Read the model definition and answer for the solid it produces. Units are mm, in the model's axes. Face numbers are marked on the shaded views. A direction names the side the tool comes from. Coordinates: 2 decimals unless noted, no trailing zeros. Order: outer loops, then holes, each group sorted by start corner. A loop starts at its lowest first (then second) coordinate and runs counter-clockwise, first axis right, second up. Notation, with made-up numbers: (74.5, 31.5) -> (97.5, 31.5) arc R34 cw to (97.5, 69.5) -> close; hole circle Ø4 at (6.25, -23). An arc over 180 degrees is marked (long way). Answer in a Markdown table with one row per item.
from build123d import *

# Parameters (mm, degrees)
F0_W     = 425.45
F0_H     = 283.972
F1_DEPTH = 101.6
F3_DEPTH = 41.275
F2_W     = 12.7
F2_H     = 69.85
F4_DEPTH = 44.45
F6_DEPTH = 12.7


with BuildPart() as f1:
    # F0 (on Top) → F1 (new body)
    with BuildSketch(Plane.XY):
        Rectangle(F0_W, F0_H)
    extrude(amount=F1_DEPTH)

    # F2 (on face) → F3 (cut)
    with BuildSketch(Plane.XY.offset(101.6)):
        with BuildLine():
            Line((104.775, 57.15), (104.775, 44.45))
            Line((104.775, 44.45), (-104.775, 44.45))
            Line((-104.775, 44.45), (-104.775, 57.15))
            Line((-104.775, 57.15), (-119.0752, 57.15))
            Line((-119.0752, 57.15), (-119.0752, 88.9))
            Line((-119.0752, 88.9), (-111.125, 88.9))
            Line((-111.125, 88.9), (-111.125, 95.25))
            Line((-111.125, 95.25), (-136.525, 95.25))
            Line((-136.525, 95.25), (-136.525, 88.9))
            Line((-136.525, 88.9), (-128.5748, 88.9))
            Line((-128.5748, 88.9), (-128.5748, 57.15))
            Line((-128.5748, 57.15), (-142.875, 57.15))
            Line((-142.875, 57.15), (-142.875, 34.925))
            Line((-142.875, 34.925), (-98.425, 34.925))
            Line((-98.425, 34.925), (-98.425, -58.3184))
            Line((-98.425, -58.3184), (-34.925, -58.3184))
            Line((-34.925, -58.3184), (0.6356468836, -93.881381557))
            Line((0.6356468836, -93.881381557), (23.5001294705, -71.0184))
            Line((23.5001294705, -71.0184), (40.6451294705, -71.0184))
            Line((40.6451294705, -71.0184), (40.6451294705, -83.7184))
            add(Edge.make_bspline(
                [(98.425, -95.25), (85.7012200048, -95.9646103609), (83.2737472807, -107.5863293593), (52.6561842817, -111.0807364969), (41.7633484197, -97.2699226213), (41.6022054851, -92.9006263614), (40.6451294705, -83.7184)],
                knots=[0, 0, 0, 0, 0.2714742221, 0.5613518333, 0.7763996456, 1, 1, 1, 1], degree=3))
            Line((98.425, -95.25), (98.425, 34.925))
            Line((98.425, 34.925), (142.875, 34.925))
            Line((142.875, 34.925), (142.875, 57.15))
            Line((142.875, 57.15), (128.5748, 57.15))
            Line((128.5748, 57.15), (128.5748, 88.9))
            Line((128.5748, 88.9), (136.525, 88.9))
            Line((136.525, 88.9), (136.525, 95.25))
            Line((136.525, 95.25), (111.125, 95.25))
            Line((111.125, 95.25), (111.125, 88.9))
            Line((111.125, 88.9), (119.0752, 88.9))
            Line((119.0752, 88.9), (119.0752, 57.15))
            Line((119.0752, 57.15), (104.775, 57.15))
        make_face()
    extrude(amount=-F3_DEPTH, mode=Mode.SUBTRACT)

    # F2 (on face) → F4 (cut)
    with BuildSketch(Plane.XY.offset(101.6)):
        with Locations((168.275, -68.961)):
            Rectangle(F2_W, F2_H)
    extrude(amount=-F4_DEPTH, mode=Mode.SUBTRACT)

    # F5 (on face) → F6 (cut)
    with BuildSketch(Plane.XY.offset(60.325)):
        Polygon((-142.875, 44.45), (-142.875, 34.925), (-98.425, 34.925), (98.425, 34.925), (142.875, 34.925), (142.875, 44.45), (104.775, 44.45), (-104.775, 44.45), align=None)
    extrude(amount=-F6_DEPTH, mode=Mode.SUBTRACT)


solid = f1.part
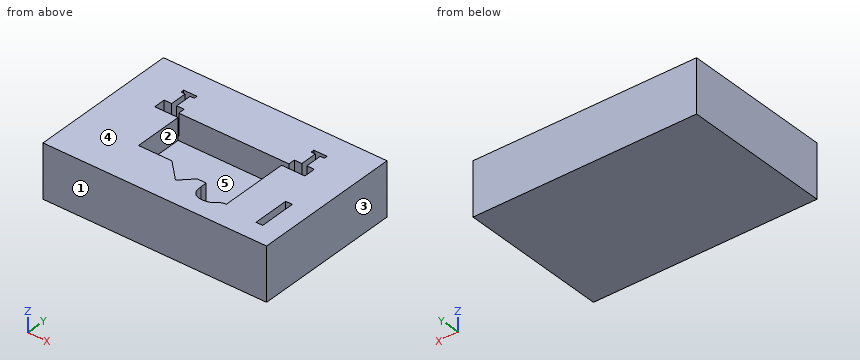
Q1. The part is cut by section B-B (x = 168.5). Write down the section's boundary in (y, z), then the cut area to 3 significant figures.
Outcome:
| item | result |
|---|---|
| outline | (-141.99, 0) -> (141.99, 0) -> (141.99, 101.6) -> (-34.04, 101.6) -> (-34.04, 57.15) -> (-103.89, 57.15) -> (-103.89, 101.6) -> (-141.99, 101.6) -> close |
| area | 25,700 mm² |
Q2. For the marked faces 4 and 5, determine the directions among +Z, -Z, +X, -X, +Y, -Y from which every point of the face is accessible in a straight line to the end or side of a thin tool.
Outcome:
| item | result |
|---|---|
| face 4 | +Z, +X, -X, +Y, -Y |
| face 5 | +Z |
Q3. Consider line 1 (X direction, y = -57, z = 80) (3 decimals); line 2 (Y direction, x = 49.5, z = 59.5) (3 decimals); line 3 (Y direction, x = -49.5, z = 72). Determine where each line is inside the solid, lowest interval first.
Outcome:
| item | result |
|---|---|
| line 1 | -212.725 to -98.425, 98.425 to 161.925, 174.625 to 212.725 |
| line 2 | -141.986 to 34.925, 44.45 to 141.986 |
| line 3 | -141.99 to -58.32, 44.45 to 141.99 |
Q4. Given pin 1 (6 mm diameter, centred on x = 58.5, y = -67.5, fed in from +Z) (3 decimals); pin 2 (4 mm diameter, centred on x = 39, y = 40.5, fed in from +Z) (3 decimals), each flat-ended and moving along its own axis, determine where each tip first touches the part or whether it passes through.
Outcome:
| item | result |
|---|---|
| pin 1 | z = 60.325 |
| pin 2 | z = 47.625 |
Q5. The part is cut by section C-C (z = 83.5). Give the number of separate pieces and of enclosed holes in the cut face, then the cut area to 3 significant figures.
Outcome:
| item | result |
|---|---|
| separate pieces | 1 |
| enclosed holes | 2 |
| area | 93,000 mm² |
Q6. The part is cut by section D-D (x = -86). Write down the section's boundary in (y, z) (3 decimals), then the cut area to 3 significant figures.
Outcome:
| item | result |
|---|---|
| outline | (-141.986, 0) -> (141.986, 0) -> (141.986, 101.6) -> (44.45, 101.6) -> (44.45, 47.625) -> (34.925, 47.625) -> (34.925, 60.325) -> (-58.318, 60.325) -> (-58.318, 101.6) -> (-141.986, 101.6) -> close |
| area | 24,500 mm² |
Q7. For a pull along X with two mould halves and no side action, classify the marked faces 1, 2 and 3 as pulls with the +X half, pulls with the -X half, needs draft (parallel to the pull), parting line crosses it, or undercut.
Outcome:
| item | result |
|---|---|
| face 1 | needs draft |
| face 2 | undercut |
| face 3 | pulls with the +X half |
Q8. The part is cut by section A-A (y = -44.5). Write down the section's boundary in (x, z) (3 decimals).
Outcome:
| item | result |
|---|---|
| outline | (-212.725, 0) -> (212.725, 0) -> (212.725, 101.6) -> (174.625, 101.6) -> (174.625, 57.15) -> (161.925, 57.15) -> (161.925, 101.6) -> (98.425, 101.6) -> (98.425, 60.325) -> (-98.425, 60.325) -> (-98.425, 101.6) -> (-212.725, 101.6) -> close |
